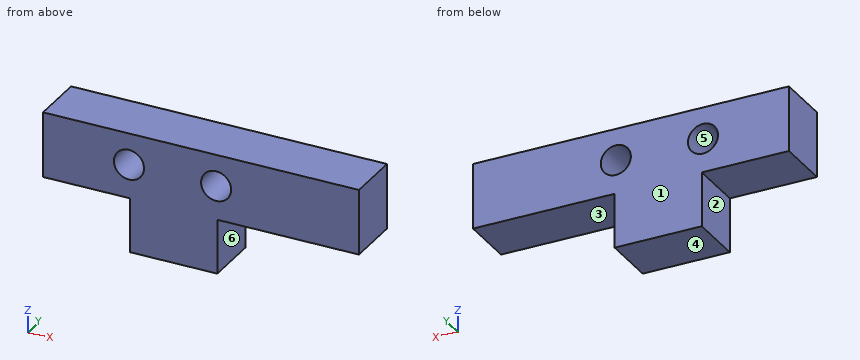
```python
from build123d import *

# Parameters (mm, degrees)
SKETCH1_W           = 30.48
SKETCH1_H           = 7.62
BOSS_EXTRUDE1_DEPTH = 3.175
SKETCH2_W           = 10.16
SKETCH2_H           = 6.35
BOSS_EXTRUDE2_DEPTH = 6.35
SKETCH3_W           = 6.35
SKETCH3_H           = 7.62
BOSS_EXTRUDE3_DEPTH = 6.35
SKETCH6_R           = 1.7526
CUT_EXTRUDE1_DEPTH  = 7.35


with BuildPart() as part:
    # Sketch1 → Boss-Extrude1 (new body, symmetric)
    with BuildSketch(Plane(origin=(0, 0, 0), x_dir=(1, 0, 0), z_dir=(0, 1, 0))):
        Rectangle(SKETCH1_W, SKETCH1_H)
    extrude(amount=BOSS_EXTRUDE1_DEPTH, both=True)

    # Sketch2 → Boss-Extrude2 (add)
    with BuildSketch(Plane(origin=(0, 3.175, 0), x_dir=(1, 0, 0), z_dir=(0, 1, 0))):
        with Locations((0, 6.985)):
            Rectangle(SKETCH2_W, SKETCH2_H)
    extrude(amount=-BOSS_EXTRUDE2_DEPTH)

    # Sketch3 → Boss-Extrude3 (add)
    with BuildSketch(Plane(origin=(0, 3.175, 0), x_dir=(1, 0, 0), z_dir=(0, 1, 0))):
        with Locations((18.415, 0)):
            Rectangle(SKETCH3_W, SKETCH3_H)
    extrude(amount=-BOSS_EXTRUDE3_DEPTH)

    # Sketch6 → Cut-Extrude1 (cut, through all)
    with BuildSketch(Plane.XZ.offset(3.175)):
        with Locations((4.941550795, 0.127)):
            Circle(SKETCH6_R)
        with Locations((-5.218449205, 0.127)):
            Circle(SKETCH6_R)
    extrude(amount=-CUT_EXTRUDE1_DEPTH, mode=Mode.SUBTRACT)


solid = part.part
```
CAD build for the part. Positions are in the model's coordinates, mm. Face numbers are marked on the shaded views. A direction names the side the tool comes from. Round coordinates to 2 decimals unless told otherwise and drop trailing zeros. Write each loop counter-clockwise with the first axis right and the second up, starting at its lowest first coordinate (ties: lowest second). Pieces come first, ordered by that corner, then holes. Notation, with made-up numbers: (38, 83) -> (73, 83) arc R12 cw to (73, 101) -> close; hole circle Ø6 at (-14, 89). An arc over 180 degrees is marked (long way). Answer in a Markdown table with one row per item. Add a question column.
Item 1: Mould opens along X. For the marked faces 4, 5 and 6 say: pulls with the +X half, pulls with the -X half, needs draft (parallel to the pull), parting line crosses it, or undercut.
Item 2: Drill centre lines: line 1 (Z direction, x = 16, y = 2.5); line 2 (X direction, y = -0.25, z = -7.25); line 3 (Z direction, x = 3.5, y = 1.25). Where is each one in solid material? Low to high. Write a range as from..to.
Item 3: Drop flat-ended pins along their axis: pin 1 Ø3 at (x, z) = (-5.22, 0.13) entering from -Y; pin 2 Ø3 at (x, y) = (-10.5, 0.5) entering from -Z. Give the stop position or say it passes through.
Item 4: Saw through at C-C, the plane z = -9. Write the cut outline in (x, y) (3 decimals), then the cut area to 3 significant figures.
Item 5: Which spindle directions (+Z, -Z, +X, -X, +Y, -Y) get a long thin tool onto all of the face, cutting with end or side? Do the marked faces 1, 2 and 3. Say none if no direction does.
Item 6: Saw through at D-D, the plane x = 15. Write the cut outline in (y, z) (3 decimals), then the cut area to 3 significant figures.
Item 7: Saw through at A-A, the plane x = -5.5. Write the cut outline in (y, z) (3 decimals), then the cut area to 3 significant figures.
Item 8: Saw through at B-B, the plane y = -2.5. Write the cut outline in (x, z).
Findings below:
| question | item | result |
|---|---|---|
| 1 | face 4 | needs draft |
| 1 | face 5 | undercut |
| 1 | face 6 | pulls with the +X half |
| 2 | line 1 | z = -3.81..3.81 |
| 2 | line 2 | x = -5.08..5.08 |
| 2 | line 3 | z = -10.16..-0.87, 1.12..3.81 |
| 3 | pin 1 | passes through |
| 3 | pin 2 | stops at z = -3.81 |
| 4 | outline | (-5.08, -3.175) -> (5.08, -3.175) -> (5.08, 3.175) -> (-5.08, 3.175) -> close |
| 4 | area | 64.5 mm^2 |
| 5 | face 1 | +Z, -Z, +X, -X, +Y |
| 5 | face 2 | -Z, -X, +Y, -Y |
| 5 | face 3 | -Z, +X, +Y, -Y |
| 6 | outline | (-3.175, -3.81) -> (3.175, -3.81) -> (3.175, 3.81) -> (-3.175, 3.81) -> close |
| 6 | area | 48.4 mm^2 |
| 7 | outline | (-3.175, -3.81) -> (3.175, -3.81) -> (3.175, -1.603) -> (-3.175, -1.603) -> close; (-3.175, 1.857) -> (3.175, 1.857) -> (3.175, 3.81) -> (-3.175, 3.81) -> close |
| 7 | area | 26.4 mm^2 |
| 8 | outline | (-15.24, -3.81) -> (-5.08, -3.81) -> (-5.08, -10.16) -> (5.08, -10.16) -> (5.08, -3.81) -> (21.59, -3.81) -> (21.59, 3.81) -> (-15.24, 3.81) -> close; hole circle Ø3.51 at (-5.22, 0.13); hole circle Ø3.51 at (4.94, 0.13) |
